```python
from build123d import *

# Parameters (mm, degrees)
SKETCH_1_W          = 6
SKETCH_1_H          = 6
EXTRUDE_1_DEPTH     = 20
HOLE_WIZARD_1_D     = 2.5
HOLE_WIZARD_1_DEPTH = 6
HOLE_WIZARD_2_D     = 2.5
HOLE_WIZARD_2_DEPTH = 6
CHAMFER_1_SIZE      = 0.3


with BuildPart() as part:
    # 草图1 → 凸台-拉伸1 (new body, symmetric)
    with BuildSketch(Plane.XY):
        Rectangle(SKETCH_1_W, SKETCH_1_H)
    extrude(amount=EXTRUDE_1_DEPTH, both=True)

    # Hole Wizard 1
    with Locations(Plane.ZY.offset(3)):
        with Locations((-15, 0), (5, 0)):
            Hole(HOLE_WIZARD_1_D / 2, depth=HOLE_WIZARD_1_DEPTH)

    # Hole Wizard 2
    with Locations(Plane(origin=(0, 3, 0), x_dir=(1, 0, 0), z_dir=(0, 1, 0))):
        with Locations((0, 5), (0, -15)):
            Hole(HOLE_WIZARD_2_D / 2, depth=HOLE_WIZARD_2_DEPTH)

    # 倒角1
    chamfer_1_edges = [part.edges().sort_by_distance(p)[0] for p in [
        (-3, 0, 20),
        (0, -3, 20),
        (3, 0, 20),
        (0, -3, -20),
        (-3, 0, -20),
        (3, 0, -20),
        (3, -3, 0),
        (-3, -3, 0),
        (-3, 3, 0),
        (3, 3, 0),
        (0, 3, 20),
    ]]
    chamfer(chamfer_1_edges, length=CHAMFER_1_SIZE)


solid = part.part
```
The listing builds one solid part. Answer for the finished solid, in the listing's coordinates (mm). Give positions to 0.01 mm unless a question says otherwise; leave off trailing zeros. Write each loop counter-clockwise with the first axis right and the second up, starting at its lowest first coordinate (ties: lowest second). Pieces come first, ordered by that corner, then holes. Notation, with made-up numbers: (86, 47) -> (140, 47) arc R35 ccw to (140, 80) -> close; hole circle Ø1 at (-32.75, 60.5). An arc over 180 degrees is marked (long way). Use one line per item in the form item = value.
1) For a pull along Y with two mould halves and no side action, classify faces 1 (the flat face through (0, 3, 0)), 2 (the cylindrical face through (0.27, -0.04, -3.78)), 3 (the cylindrical face through (0.04, 0.05, -13.75)), 4 (the flat face through (0, -3, 0)) as +Y half, -Y half, draft (parallel to the pull), parting line (faces both ways), or undercut.
Result:
face_1 = +Y half
face_2 = draft
face_3 = undercut
face_4 = -Y half
2) Section D-D on y = 2 is taken. Write down the section's boundary in (x, z), plus the area to 3 significant figures.
Result:
outline = (-3, -19.7) -> (-2.7, -20) -> (2.7, -20) -> (3, -19.7) -> (3, 19.7) -> (2.7, 20) -> (-2.7, 20) -> (-3, 19.7) -> close; hole circle Ø2.5 at (0, -5); hole circle Ø2.5 at (0, 15)
area = 230 mm²
3) Straight lines are drawn through the part: probe 1 along Z at (x, y) = (-0.25, 0.5); probe 2 along Y at (x, z) = (1.15, -15); probe 3 along Z at (x, y) = (-1, 2.75). For each, find the intervals that lie inside material, in ascending order.
Result:
probe_1 = -20 to -16.15, -13.85 to -6.22, -3.78 to 3.85, 6.15 to 13.78, 16.22 to 20
probe_2 = -3 to -1.25, 1.25 to 3
probe_3 = -20 to -5.75, -4.25 to 14.25, 15.75 to 19.95
4) Section C-C on z = -5 is taken. Write down the section's boundary in (x, y).
Result:
outline = (-3, -2.7) -> (-2.7, -3) -> (-1.25, -3) -> (-1.25, 3) -> (-2.7, 3) -> (-3, 2.7) -> close; (1.25, -3) -> (2.7, -3) -> (3, -2.7) -> (3, 2.7) -> (2.7, 3) -> (1.25, 3) -> close
5) Section A-A on x = 0.75 is taken. Write down the section's boundary in (y, z), plus the area to 3 significant figures.
Result:
outline = (-3, -19.7) -> (-2.7, -20) -> (3, -20) -> (3, -6) -> (-3, -6) -> close; (-3, -4) -> (3, -4) -> (3, 14) -> (-3, 14) -> close; (-3, 16) -> (3, 16) -> (3, 19.7) -> (2.7, 20) -> (-2.7, 20) -> (-3, 19.7) -> close; hole circle Ø2.5 at (0, -15); hole circle Ø2.5 at (0, 5)
area = 206 mm²
6) Section B-B on y = 0 is taken. Write down the section's boundary in (x, z).
Result:
outline = (-3, -19.7) -> (-2.7, -20) -> (2.7, -20) -> (3, -19.7) -> (3, -16.25) -> (-3, -16.25) -> close; (-3, -13.75) -> (3, -13.75) -> (3, 3.75) -> (-3, 3.75) -> close; (-3, 6.25) -> (3, 6.25) -> (3, 19.7) -> (2.7, 20) -> (-2.7, 20) -> (-3, 19.7) -> close; hole circle Ø2.5 at (0, -5); hole circle Ø2.5 at (0, 15)
